For this review, take the finished solid that the model builds, in its own axes (mm). A direction names the side the tool comes from. Coordinates: 2 decimals unless noted, no trailing zeros. Loops run counter-clockwise (first coordinate to the right, second up) from the corner with the lowest first, then second, coordinate; pieces in that order, holes last. Notation, with made-up numbers: (-5, 39.5) -> (16, 39.5) arc R25 cw to (16, 63.5) -> close; hole circle Ø4 at (-40, 43.5). An arc over 180 degrees is marked (long way). Answer in a Markdown table with one row per item.
from build123d import *

# Parameters (mm, degrees)
BOSS_EXTRU_1_DEPTH                      = 6
ESQUISSE2_R                             = 2.5
ENL_V_MAT_EXTRU_1_DEPTH                 = 6
CHANFREIN1_SIZE                         = 5
ESQUISSE6_W                             = 29.69
ESQUISSE6_H                             = 3
ENL_VEMENT_DE_MATI_RE_R_VOLUTION1_ANGLE = 1
ESQUISSE7_W                             = 3
ESQUISSE7_H                             = 29.29
R_VOLUTION2_ANGLE                       = 1
ENL_V_MAT_EXTRU_2_DEPTH                 = 10


with BuildPart() as part:
    # Esquisse1 → Boss.-Extru.1 (new body)
    with BuildSketch(Plane.XY):
        with BuildLine():
            Line((0, 277.3), (0, 239.61))
            ThreePointArc((0, 239.61), (119.805, 207.508347001), (207.508347001, 119.805))
            Line((207.508347001, 119.805), (240.148844469, 138.65))
            ThreePointArc((240.148844469, 138.65), (138.65, 240.148844469), (0, 277.3))
        make_face()
    extrude(amount=BOSS_EXTRU_1_DEPTH)

    # Esquisse2 → Enlèv. mat.-Extru.1 (cut)
    with BuildSketch(Plane.XY.offset(6)):
        with Locations((67.155777633, 250.628774147)):
            Circle(ESQUISSE2_R)
        with Locations((109.656760374, 235.159681502)):
            Circle(ESQUISSE2_R)
        with Locations((212.545380932, 148.82587794)):
            Circle(ESQUISSE2_R)
        with Locations((183.472996514, 183.472996514)):
            Circle(ESQUISSE2_R)
    extrude(amount=-ENL_V_MAT_EXTRU_1_DEPTH, mode=Mode.SUBTRACT)

    # Chanfrein1
    chanfrein1_edges = [part.edges().sort_by_distance(p)[0] for p in [
        (64.655777633, 250.628774147, 6),
        (107.156760374, 235.159681502, 6),
        (180.972996514, 183.472996514, 6),
        (210.045380932, 148.82587794, 6),
    ]]
    chamfer(chanfrein1_edges, length=CHANFREIN1_SIZE)

    # Esquisse6 → Enlèvement de matière-Révolution1 (revolve, cut)
    with BuildSketch(Plane(origin=(0, 0, 0), x_dir=(0.8660254037844394, 0.49999999999999883, 0), z_dir=(0.49999999999999883, -0.8660254037844394, 0))):
        with Locations((258.455, 4.5)):
            Rectangle(ESQUISSE6_W, ESQUISSE6_H)
    revolve(axis=Axis((0, 0, 0), (0, 0, 1)), revolution_arc=ENL_VEMENT_DE_MATI_RE_R_VOLUTION1_ANGLE, mode=Mode.SUBTRACT)

    # Esquisse7 → Révolution2 (revolve)
    with BuildSketch(Plane.ZY):
        with Locations((4.5, 258.455)):
            Rectangle(ESQUISSE7_W, ESQUISSE7_H)
    revolve(axis=Axis((0, 0, 0), (0, 0, 1)), revolution_arc=R_VOLUTION2_ANGLE)

    # Esquisse8 → Enlèv. mat.-Extru.2 (cut)
    with BuildSketch(Plane.XY.offset(6)):
        Polygon((-4.291451908, 245.857115173), (-0.980595059, 243.808028033), (-4.255071213, 243.772866556), align=None)
    extrude(amount=-ENL_V_MAT_EXTRU_2_DEPTH, mode=Mode.SUBTRACT)


solid = part.part
Item 1: Insertion check: pin 1 (1.8 mm diameter, centred on y = 261, z = 2.5, fed in from -X); pin 2 (2 mm diameter, centred on x = 90.5, z = 5.5, fed in from +Y); pin 3 (8 mm diameter, centred on x = 183.47, y = 183.47, fed in from +Z). Each pin has a flat end and moves straight along its axis. Give the tip position at first contact, or say it passes through.
Worked answers:
| item | result |
|---|---|
| pin 1 | x = -4.57 |
| pin 2 | y = 262.46 |
| pin 3 | z = 2.5 |
Item 2: For L1, parallel to Y at x = 186, z = 2.8; L2, parallel to Y at x = 212, z = 2.4; L3, parallel to X at y = 218, z = 4.8, list the stretches that pass through material, from the lowest coordinate up.
Worked answers:
| item | result |
|---|---|
| L1 | 151.05 to 179.99, 186.95 to 205.67 |
| L2 | 122.4 to 144.96, 152.69 to 178.75 |
| L3 | 99.44 to 171.38 |
Item 3: Take a section at B-B, the plane x = 168. State the section outline as (y, z) points, and give its area (3 significant figures).
Worked answers:
| item | result |
|---|---|
| outline | (170.85, 0) -> (220.62, 0) -> (220.62, 6) -> (170.85, 6) -> close |
| area | 299 mm² |
Item 4: For faces 4 (the conical face through (66.561, 247.951, 1.243)), 5 (the flat face through (-2, 259, 3)), list the 3-axis set-ups (+Z, -Z, +X, -X, +Y, -Y) from which the entire face can be reached by the end or side of a thin tool; tool diameter is ignored.
Worked answers:
| item | result |
|---|---|
| face 4 | +Z |
| face 5 | -Z, -X, +Y, -Y |
Item 5: Take a section at C-C, the plane x = 87. State the section outline as (y, z) points.
Worked answers:
| item | result |
|---|---|
| outline | (223.26, 0) -> (263.3, 0) -> (263.3, 6) -> (223.26, 6) -> close |
Item 6: The part is to be moulded in two halves that separate along X. For faces 1 (the cylindrical face through (140.407, 239.126, 2.958)), 2 (the conical face through (184.739, 181.04, 1.243)), 3 (the flat face through (120, 216, 0)), say which applies: +X half, -X half, draft (parallel to the pull), parting line (faces both ways), or undercut.
Worked answers:
| item | result |
|---|---|
| face 1 | +X half |
| face 2 | undercut |
| face 3 | draft |
Item 7: Take a section at A-A, the plane z = 4.5. State the section outline as (x, y) points (3 decimals).
Worked answers:
| item | result |
|---|---|
| outline | (-4.766, 273.058) -> (-4.291, 245.857) -> (-0.981, 243.808) arc R243.81 cw to (0, 243.81) -> (0, 239.61) arc R239.61 cw to (207.508, 119.805) -> (210.972, 121.805) arc R243.61 ccw to (208.815, 125.468) -> (234.264, 140.76) arc R273.3 cw to (236.685, 136.65) -> (240.149, 138.65) arc R277.3 ccw to (0, 277.3) -> (0, 273.1) arc R273.1 ccw to start; hole circle Ø12 at (67.156, 250.629); hole circle Ø12 at (109.657, 235.16); hole circle Ø12 at (183.473, 183.473); hole circle Ø12 at (212.545, 148.826) |
